from build123d import *

# Parameters (mm, degrees)
CROQUIS1_R              = 50
CROQUIS1_R_2            = 3.4
CROQUIS1_R_3            = 4
SALIENTE_EXTRUIR1_DEPTH = 10


with BuildPart() as part:
    # Croquis1 → Saliente-Extruir1 (new body)
    with BuildSketch(Plane(origin=(0, 0, 0), x_dir=(1, 0, 0), z_dir=(0, 1, 0))):
        with BuildLine():
            Line((-99.733333333, 137.670847394), (-222.7, 48.589710845))
            ThreePointArc((-222.7, 48.589710845), (-247.5, 0), (-222.7, -48.589710845))
            Line((-222.7, -48.589710845), (-99.733333333, -137.670847394))
            ThreePointArc((-99.733333333, -137.670847394), (0, -170), (99.733333333, -137.670847394))
            Line((99.733333333, -137.670847394), (222.7, -48.589710845))
            ThreePointArc((222.7, -48.589710845), (247.5, 0), (222.7, 48.589710845))
            Line((222.7, 48.589710845), (99.733333333, 137.670847394))
            ThreePointArc((99.733333333, 137.670847394), (0, 170), (-99.733333333, 137.670847394))
        make_face()
        Circle(CROQUIS1_R, mode=Mode.SUBTRACT)
        with Locations((-95, 70)):
            Circle(CROQUIS1_R_2, mode=Mode.SUBTRACT)
        with Locations((95, 70)):
            Circle(CROQUIS1_R_2, mode=Mode.SUBTRACT)
        with Locations((95, -70)):
            Circle(CROQUIS1_R_2, mode=Mode.SUBTRACT)
        with Locations((-95, -70)):
            Circle(CROQUIS1_R_2, mode=Mode.SUBTRACT)
        with Locations((187.5, 0)):
            Circle(CROQUIS1_R_3, mode=Mode.SUBTRACT)
        with Locations((-187.5, 0)):
            Circle(CROQUIS1_R_3, mode=Mode.SUBTRACT)
    extrude(amount=SALIENTE_EXTRUIR1_DEPTH)


solid = part.part
Here's how the part is built. I have some questions about the finished solid (model axes, mm). Give positions to 0.01 mm unless a question says otherwise; leave off trailing zeros. Loops run counter-clockwise (first coordinate to the right, second up) from the corner with the lowest first, then second, coordinate; pieces in that order, holes last. Notation, with made-up numbers: (-5.75, -39) -> (50.25, -39) arc R23 ccw to (50.25, -27) -> close; hole circle Ø2 at (77, 19). An arc over 180 degrees is marked (long way). One line per item, written item: value.
Q1. Suppose I cut it at B-B on y = 6. Please give me the cut outline in (x, z).
Answers follow:
outline: (-222.7, -48.59) -> (-99.73, -137.67) arc R170 ccw to (99.73, -137.67) -> (222.7, -48.59) arc R60 ccw to (222.7, 48.59) -> (99.73, 137.67) arc R170 ccw to (-99.73, 137.67) -> (-222.7, 48.59) arc R60 ccw to start; hole circle Ø8 at (-187.5, 0); hole circle Ø6.8 at (-95, -70); hole circle Ø6.8 at (-95, 70); hole circle Ø100 at (0, 0); hole circle Ø6.8 at (95, -70); hole circle Ø6.8 at (95, 70); hole circle Ø8 at (187.5, 0)
Q2. Suppose I cut it at D-D on x = 110. Please give me the cut outline in (y, z), then the cut area to 3 significant figures.
Answers follow:
outline: (0, -130.23) -> (10, -130.23) -> (10, 130.23) -> (0, 130.23) -> close
area: 2,600 mm^2
Q3. I'm going to push flat-ended pins straight in: pin 1 Ø4 at (x, z) = (95, 70) entering from +Y; pin 2 Ø4 at (y, z) = (5, 63.5) entering from +X; pin 3 Ø1 at (x, y) = (-153, 8.5) entering from +Z; pin 4 Ø5 at (y, z) = (2, 13.5) entering from -X. Where does each tip first touch, or does it pass through?
Answers follow:
pin 1: through
pin 2: x = 204.88
pin 3: z = 99.44
pin 4: x = -246.48
Q4. Suppose I cut it at A-A on x = 0. Please give me the cut outline in (y, z), then the cut area to 3 significant figures.
Answers follow:
outline: (0, -170) -> (10, -170) -> (10, -50) -> (0, -50) -> close; (0, 50) -> (10, 50) -> (10, 170) -> (0, 170) -> close
area: 2,400 mm^2
Q5. Suppose I cut it at C-C on z = 103. Please give me the cut outline in (x, y).
Answers follow:
outline: (-147.59, 0) -> (147.59, 0) -> (147.59, 10) -> (-147.59, 10) -> close
Q6. We'd pull the mould along Z, two halves only. Please class faces 1 (the face through (47.69, 4.93, -15.02)), 2 (the face through (-58, 10, -2)), 3 (the face through (1.492, 4.93, -169.993)): pulls with the +Z half, pulls with the -Z half, needs draft (parallel to the pull), parting line crosses it, or undercut.
Answers follow:
face 1: undercut
face 2: needs draft
face 3: pulls with the -Z half
Q7. If I drill on line 1 along X through (y, z) = (2.5, 0); line 2 along Z through (x, y) = (-95, 5); line 3 along X through (y, z) = (7.25, -70), over which ranges is the centre line in solid material (lowest first)?
Answers follow:
line 1: -247.5 to -191.5, -183.5 to -50, 50 to 183.5, 191.5 to 247.5
line 2: -140.98 to -73.4, -66.6 to 66.6, 73.4 to 140.98
line 3: -193.15 to -98.4, -91.6 to 91.6, 98.4 to 193.15
